Autodesk Inventor part; units mm, degrees
ref_plane "YZ Plane" through (0, 0, 0) normal (1, 0, 0) x (0, 1, 0)
ref_plane "XZ Plane" through (0, 0, 0) normal (0, 1, 0) x (-1, 0, 0)
ref_plane "XY Plane" through (0, 0, 0) normal (0, 0, 1) x (1, 0, 0)
sketch "スケッチ1" plane through (0, 0, 0) normal (0, 0, 1) x (1, 0, 0)
  line L0 (-12.5, 25) -> (12.5, 25)
  line L1 (12.5, 25) -> (12.5, -25)
  line L2 (12.5, -25) -> (-12.5, -25)
  line L3 (-12.5, -25) -> (-12.5, 25)
  line L4 (-10.5, 25) -> (10.5, 25)
  line L5 (10.5, 25) -> (10.5, -23)
  line L6 (10.5, -23) -> (-10.5, -23)
  line L7 (-10.5, -23) -> (-10.5, 25)
  point P0 (0, 0)
  dimension "d0" = 25
  dimension "d1" = 50
  dimension "d2" = 25
  dimension "d3" = 12.5
  dimension "d4" = 2
  dimension "d5" = 2
  dimension "d6" = 2
extrude "押し出し1" add sketch "スケッチ1" along normal blind 60 contours L0 L7 L6 L5 L1 L2 L3
sketch "スケッチ2" plane through (12.5, -25, 0) normal (1, 0, 0) x (0, 0, -1)
  line L0 (0, 50) -> (-60, 50)
  line L1 (-30, 50) -> (-30, 0)
  line L2 (0, 0) -> (-60, 0)
  line L3 (-60, 50) -> (-60, 0)
  point P0 (0, 25)
  point P1 (-52, 42)
  point P2 (-32, 42)
  dimension "d11" = 8
  dimension "d12" = 8
  dimension "d76" = 8
  dimension "d84" = 20
hole "Hole1" at (12.5, 17, 52) at (12.5, 17, 32) direction (-1, 0, 0) diameter 6 end through all
sketch "スケッチ5" plane through (-12.5, -25, 0) normal (0, -1, 0) x (1, 0, 0)
  line L0 (25, 60) -> (0, 60)
  line L1 (25, 0) -> (25, 60)
  line L2 (12.5, 60) -> (12.5, 0)
  line L3 (0, 0) -> (25, 0)
  point P0 (4.8, 34.096)
  point P1 (5.3, 2.996)
  point P2 (19.7, 3)
  point P3 (20.2, 34.1)
  dimension "d46" = 14.4
  dimension "d47" = 15.4
  dimension "d48" = 31.1
  dimension "d50" = 15.4
  dimension "d51" = 14.4
  dimension "d52" = 31.1
  dimension "d53" = 3
hole "Hole3" at (-7.7, -25, 34.096) at (-7.2, -25, 2.996) at (7.2, -25, 3) at (7.7, -25, 34.1) direction (0, 1, 0) diameter 2.5 end through all
sketch "スケッチ6" plane through (-12.5, -25, 0) normal (0, -1, 0) x (1, 0, 0)
  circle A0 centre (5.3, 2.996) radius 1.25
  point P0 (12.5, 0)
  point P1 (12.5, 9.196)
  dimension "d54" = 7.2
  dimension "d55" = 6.2
hole "Hole4" at (0, -25, 9.196) direction (0, 1, 0) diameter 10 depth 8 tip angle 118
sketch "スケッチ7" plane through (-12.5, -25, 0) normal (0, -1, 0) x (1, 0, 0)
  circle A0 centre (4.8, 34.096) radius 1.25
  line L0 (25, 60) -> (0, 60)
  line L1 (0, 0) -> (25, 0)
  line L2 (2.5, 32.096) -> (22.5, 32.096)
  line L3 (22.5, 32.096) -> (22.5, 16.096)
  line L4 (22.5, 16.096) -> (2.5, 16.096)
  line L5 (2.5, 16.096) -> (2.5, 32.096)
  line L6 (12.5, 60) -> (12.5, 0)
  dimension "d63" = 16
  dimension "d64" = 20
  dimension "d65" = 20
  dimension "d66" = 2
extrude "押し出し3" cut sketch "スケッチ7" against normal through all contours L2 L6 L4 L5 | L2 L3 L4 L6
fillet "フィレット3" radius 5 2 edges at (-10, -24, 16.096) (10, -24, 16.096)
fillet "フィレット4" radius 1 2 edges at (-10, -24, 32.096) (10, -24, 32.096)
sketch "スケッチ9" plane through (12.5, -25, 0) normal (1, 0, 0) x (0, 0, -1)
  circle A0 centre (-32, 42) radius 3
  line L0 (0, 50) -> (-24, 50)
  line L1 (-24, 50) -> (-24, 24)
  line L2 (-24, 24) -> (0, 24)
  line L3 (0, 24) -> (0, 50)
  line L4 (0, 2) -> (-60, 2)
  point P0 (0, 25)
  dimension "d77" = 8
  dimension "d78" = 22
extrude "押し出し5" cut sketch "スケッチ9" against normal through all contours L3 L2 L1 L0
fillet "フィレット5" radius 3 2 edges at (11.5, -1, 24) (-11.5, -1, 24)
fillet "フィレット6" radius 8 4 edges at (-11.5, 25, 60) (11.5, 25, 60) (11.5, 25, 24) (-11.5, 25, 24)
fillet "フィレット7" radius 3 2 edges at (11.5, -1, 0) (-11.5, -1, 0)
equation "\"d1\" = 2 * d0"
equation "\"d4\" = d5"
equation "\"d6\" = d5"
equation "\"d65\" = d64"
properties part number "JointC3"
Geometry check sheet. Reference: the model listing, model coordinates, mm. A direction names the side the tool comes from. Round coordinates to 2 decimals unless told otherwise and drop trailing zeros. Loops run counter-clockwise (first coordinate to the right, second up) from the corner with the lowest first, then second, coordinate; pieces in that order, holes last. Notation, with made-up numbers: (81.25, 34) - (121.25, 34) arc R26 ccw to (121.25, 57) - close; hole circle Ø7 at (7, 87.25). An arc over 180 degrees is marked (long way). Write item = value, one per line. Start each with the question number.
1. Section check D-D on y = 16. Enter the section's corners in (x, z).
2. Section check A-A on x = 0. Enter the section's corners in (y, z).
3. Section check B-B on y = -7.5. Enter the section's corners in (x, z), then the cut area to 3 significant figures.
4. Thickness scan on line 1 (Z direction, x = 11.2, y = 17); line 2 (X direction, y = -16.5, z = 3); line 3 (Z direction, x = -7.2, y = -24.35). Record the ranges inside material, lowest first.
5. Section check C-C on z = 34.1. Enter the section's corners in (x, y), then the cut area to 3 significant figures.
6. Set-up check for faces 5 (the face through (0, -24, 32.096)), 6 (the face through (-11, -9, 60)), 7 (the face through (-11, -1, 12)), 8 (the face through (-12, 17, 55)), 9 (the face through (-10.5, -5, 36)): record each of +Z, -Z, +X, -X, +Y, -Y from which the full face is reachable in a straight line by a thin tool's end or side.
7. Mould release check, pull along Y, two halves, no side actions. Record for faces 1 (the face through (11.514, 22.719, 57.594)), 2 (the face through (12.5, -5, 36)), 3 (the face through (0, -25, 36)), 4 (the face through (-12, 17, 35)): released by +Y, released by -Y, zero draft, split by the parting line, or undercut.
8. Depth check by flat-ended pin: pin 1 (3 mm diameter, centred on x = 9.5, z = 17, fed in from +Y); pin 2 (1 mm diameter, centred on x = 11.5, y = 9, fed in from -Z). Enter the tip coordinate at first touch or a pass-through.
Working result:
q1.outline = (-12.5, 24) - (-10.5, 24) - (-10.5, 29.17) - (-12.5, 29.17) - close; (-12.5, 34.83) - (-10.5, 34.83) - (-10.5, 49.17) - (-12.5, 49.17) - close; (-12.5, 54.83) - (-10.5, 54.83) - (-10.5, 60) - (-12.5, 60) - close; (10.5, 24) - (12.5, 24) - (12.5, 29.17) - (10.5, 29.17) - close; (10.5, 34.83) - (12.5, 34.83) - (12.5, 49.17) - (10.5, 49.17) - close; (10.5, 54.83) - (12.5, 54.83) - (12.5, 60) - (10.5, 60) - close
q2.outline = (-25, 0) - (-23, 0) - (-23, 4.2) - (-25, 4.2) - close; (-25, 14.2) - (-23, 14.2) - (-23, 16.1) - (-25, 16.1) - close; (-25, 32.1) - (-23, 32.1) - (-23, 60) - (-25, 60) - close
q3.outline = (-12.5, 0) - (-10.5, 0) - (-10.5, 60) - (-12.5, 60) - close; (10.5, 0) - (12.5, 0) - (12.5, 60) - (10.5, 60) - close
q3.area = 240 mm^2
q4.line_1 = 24 to 29, 35 to 49, 55 to 60
q4.line_2 = -12.5 to -10.5, 10.5 to 12.5
q4.line_3 = 0 to 1.75, 4.25 to 16.61, 32.1 to 32.95, 35.24 to 60
q5.outline = (-12.5, -25) - (-8.95, -25) - (-8.95, -23) - (-10.5, -23) - (-10.5, 14.86) - (-12.5, 14.86) - close; (-12.5, 19.14) - (-10.5, 19.14) - (-10.5, 25) - (-12.5, 25) - close; (-6.45, -25) - (6.45, -25) - (6.45, -23) - (-6.45, -23) - close; (8.95, -25) - (12.5, -25) - (12.5, 14.86) - (10.5, 14.86) - (10.5, -23) - (8.95, -23) - close; (10.5, 19.14) - (12.5, 19.14) - (12.5, 25) - (10.5, 25) - close
q5.area = 215 mm^2
q6.face_5 = +Y, -Y
q6.face_6 = +Z, +X, -X, +Y, -Y
q6.face_7 = -Z, +X, -X, +Y
q6.face_8 = +X, -X
q6.face_9 = +Z, -Z, +Y
q7.face_1 = released by +Y
q7.face_2 = zero draft
q7.face_3 = released by -Y
q7.face_4 = undercut
q8.pin_1 = -1
q8.pin_2 = 24
